```python
from build123d import *

# Parameters (mm, degrees)
SKETCH_1_W      = 10
SKETCH_1_H      = 3
EXTRUDE_3_DEPTH = 3


with BuildPart() as part:
    # 草图1 → 凸台-拉伸3 (new body)
    with BuildSketch(Plane.XY):
        Polygon((-37, 5), (-37, -5), (-37, -10), (37, -10), (37, -5), (37, 5), (37, 10), (-37, 10), align=None)
        with Locations((-15, 6.5)):
            Rectangle(SKETCH_1_W, SKETCH_1_H, mode=Mode.SUBTRACT)
        with Locations((-30, 6.5)):
            Rectangle(SKETCH_1_W, SKETCH_1_H, mode=Mode.SUBTRACT)
        with Locations((0, 6.5)):
            Rectangle(SKETCH_1_W, SKETCH_1_H, mode=Mode.SUBTRACT)
        with Locations((15, 6.5)):
            Rectangle(SKETCH_1_W, SKETCH_1_H, mode=Mode.SUBTRACT)
        with Locations((30, 6.5)):
            Rectangle(SKETCH_1_W, SKETCH_1_H, mode=Mode.SUBTRACT)
        with Locations((30, -6.5)):
            Rectangle(SKETCH_1_W, SKETCH_1_H, mode=Mode.SUBTRACT)
        with Locations((15, -6.5)):
            Rectangle(SKETCH_1_W, SKETCH_1_H, mode=Mode.SUBTRACT)
        with Locations((0, -6.5)):
            Rectangle(SKETCH_1_W, SKETCH_1_H, mode=Mode.SUBTRACT)
        with Locations((-15, -6.5)):
            Rectangle(SKETCH_1_W, SKETCH_1_H, mode=Mode.SUBTRACT)
        with Locations((-30, -6.5)):
            Rectangle(SKETCH_1_W, SKETCH_1_H, mode=Mode.SUBTRACT)
    extrude(amount=EXTRUDE_3_DEPTH)


solid = part.part
```
Check sheet for the modelled part. Datum: model origin and axes. Units: mm. A direction names the side the tool comes from. Coordinates: 2 decimals unless noted, no trailing zeros. Write each loop counter-clockwise with the first axis right and the second up, starting at its lowest first coordinate (ties: lowest second). Pieces come first, ordered by that corner, then holes. Notation, with made-up numbers: M -9,21.5 L 35,21.5 A20 cw 35,49.5 Z; hole C 60.5,-39 d9. An arc over 180 degrees is marked long. Write item = value, one per line. Start each with the question number.
1. Tool access check on faces 1 (the flat face through (-35, -7, 1)), 2 (the flat face through (-1, -10, 1)). Record the directions out of +Z, -Z, +X, -X, +Y, -Y that give a thin tool (end or side, any length) a straight path to the whole face; none if there is none.
2. Sectioned sample at C-C (z = 0.8). State how many separate pieces and enclosed holes the cut face has, then the cut area to 3 significant figures.
3. Sectioned sample at B-B (x = -17.5). Record the cut outline in (y, z), then the cut area to 3 significant figures.
4. Mould release check, pull along X, two halves, no side actions. Record for faces 3 (the flat face through (-1, 0, 3)), 4 (the flat face through (-25, -7, 1)), 5 (the flat face through (25, 6, 1)): pulls with the +X half, pulls with the -X half, needs draft (parallel to the pull), parting line crosses it, or undercut.
5. Thickness scan on probe 1 along X at (y, z) = (-5.75, 1.65); probe 2 along Y at (x, z) = (-33, 1.6). Record the ranges inside material, lowest first.
6. Sectioned sample at A-A (y = 6.75). Record the cut outline in (x, z).
The answers:
q1.face_1 = +Z, -Z
q1.face_2 = +Z, -Z, +X, -X, -Y
q2.separate_pieces = 1
q2.enclosed_holes = 10
q2.area = 1,180 mm²
q3.outline = M -10,0 L -8,0 L -8,3 L -10,3 Z; M -5,0 L 5,0 L 5,3 L -5,3 Z; M 8,0 L 10,0 L 10,3 L 8,3 Z
q3.area = 42.0 mm²
q4.face_3 = needs draft
q4.face_4 = undercut
q4.face_5 = undercut
q5.probe_1 = -37 to -35, -25 to -20, -10 to -5, 5 to 10, 20 to 25, 35 to 37
q5.probe_2 = -10 to -8, -5 to 5, 8 to 10
q6.outline = M -37,0 L -35,0 L -35,3 L -37,3 Z; M -25,0 L -20,0 L -20,3 L -25,3 Z; M -10,0 L -5,0 L -5,3 L -10,3 Z; M 5,0 L 10,0 L 10,3 L 5,3 Z; M 20,0 L 25,0 L 25,3 L 20,3 Z; M 35,0 L 37,0 L 37,3 L 35,3 Z
